Check sheet for the modelled part. Datum: model origin and axes. Units: mm. A direction names the side the tool comes from. Round coordinates to 2 decimals unless told otherwise and drop trailing zeros. Write each loop counter-clockwise with the first axis right and the second up, starting at its lowest first coordinate (ties: lowest second). Pieces come first, ordered by that corner, then holes.
Item 1: Release check for a two-part mould opening along Z. For faces 1 (the cylindrical face through (3.143, -71.896, 28.193)), 2 (the flat face through (12, -44, 0)), 3 (the cylindrical face through (23, -1, 3)) record: pulls with the +Z half, pulls with the -Z half, needs draft (parallel to the pull), parting line crosses it, or undercut.
Item 2: Section check D-D, the plane y = -23. Record the cut outline in (x, z), plus the area to 3 significant figures.
Item 3: Depth check by flat-ended pin: pin 1 (1.5 mm diameter, centred on x = 2.5, z = 17, fed in from +Y); pin 2 (3 mm diameter, centred on y = -53, z = 26.5, fed in from +X); pin 3 (2.5 mm diameter, centred on y = -55, z = 9, fed in from +X); pin 4 (6.5 mm diameter, centred on x = 11, y = -40, fed in from +Z). Enter the tip coordinate at first touch or a pass-through.
Item 4: Section check B-B, the plane y = -67.5. Record the cut outline in (x, z).
Item 5: Material ranges on line 1 along Z through (x, y) = (3.75, -22.5); line 2 along Z through (x, y) = (1.75, -67.5); line 3 along Z through (x, y) = (5.75, -21), recorded low to high.
Item 6: Section check C-C, the plane x = 2. Record the cut outline in (y, z).
Item 7: Section check A-A, the plane z = 28. Record the cut outline in (x, y), plus the area to 3 significant figures.
Item 8: Set-up check for faces 4 (the flat face through (6.2, -44, 24)), 5 (the flat face through (0, -44, 19)), 6 (the flat face through (5, -46, 11.2)): record each of +Z, -Z, +X, -X, +Y, -Y from which the full face is reachable in a straight line by a thin tool's end or side.
from build123d import *

# Parameters (mm, degrees)
F1_DEPTH = 90
F3_D     = 8.8
F4_R     = 5
F5_W     = 3
F5_H     = 5
F6_DEPTH = 90


with BuildPart() as f1:
    # F0 (on Front) → F1 (new body)
    with BuildSketch(Plane.XZ):
        Polygon((0, 38), (0, 0), (25, 0), (25, 6.2), (6.2, 6.2), (6.2, 38), align=None)
    extrude(amount=F1_DEPTH)

    # F3 (through all)
    with Locations(Plane(origin=(0, 0, 0), x_dir=(0, -1, 0), z_dir=(-1, 0, 0))):
        with Locations((67.5, 28), (22.5, 28)):
            Hole(F3_D / 2)

    # F4
    f4_edges = [f1.edges().sort_by_distance(p)[0] for p in [
        (25, -90, 3.1),
        (25, 0, 3.1),
    ]]
    fillet(f4_edges, radius=F4_R)

    # F5 (on face) → F6 (cut)
    with BuildSketch(Plane.XZ.offset(90)):
        with Locations((4.7, 8.7)):
            Rectangle(F5_W, F5_H)
    extrude(amount=-F6_DEPTH, mode=Mode.SUBTRACT)


solid = f1.part
Values found:
1. face 1: undercut
1. face 2: pulls with the -Z half
1. face 3: needs draft
2. outline: (0, 0) - (25, 0) - (25, 6.2) - (3.2, 6.2) - (3.2, 11.2) - (6.2, 11.2) - (6.2, 23.63) - (0, 23.63) - close; (0, 32.37) - (6.2, 32.37) - (6.2, 38) - (0, 38) - close
2. area: 283 mm2
3. pin 1: stops at y = 0
3. pin 2: stops at x = 6.2
3. pin 3: stops at x = 3.2
3. pin 4: stops at z = 6.2
4. outline: (0, 0) - (25, 0) - (25, 6.2) - (3.2, 6.2) - (3.2, 11.2) - (6.2, 11.2) - (6.2, 23.6) - (0, 23.6) - close; (0, 32.4) - (6.2, 32.4) - (6.2, 38) - (0, 38) - close
5. line 1: z = 0 to 6.2, 11.2 to 23.6, 32.4 to 38
5. line 2: z = 0 to 23.6, 32.4 to 38
5. line 3: z = 0 to 6.2, 11.2 to 23.86, 32.14 to 38
6. outline: (-90, 0) - (0, 0) - (0, 38) - (-90, 38) - close; hole circle Ø8.8 at (-67.5, 28); hole circle Ø8.8 at (-22.5, 28)
7. outline: (0, -90) - (6.2, -90) - (6.2, -71.9) - (0, -71.9) - close; (0, -63.1) - (6.2, -63.1) - (6.2, -26.9) - (0, -26.9) - close; (0, -18.1) - (6.2, -18.1) - (6.2, 0) - (0, 0) - close
7. area: 449 mm2
8. face 4: +Z, +X, +Y, -Y
8. face 5: +Z, -Z, -X, +Y, -Y
8. face 6: +X, +Y, -Y
